from build123d import *

# Parameters (mm, degrees)
SKETCH1_W           = 20
SKETCH1_H           = 24
BOSS_EXTRUDE1_DEPTH = 8
SKETCH2_R           = 7
CUT_EXTRUDE1_DEPTH  = 22
BOSS_EXTRUDE2_DEPTH = 2


with BuildPart() as part:
    # Sketch1 → Boss-Extrude1 (new body)
    with BuildSketch(Plane(origin=(0, 0, 0), x_dir=(1, 0, 0), z_dir=(0, 1, 0))):
        Rectangle(SKETCH1_W, SKETCH1_H)
    extrude(amount=BOSS_EXTRUDE1_DEPTH)

    # Sketch2 → Cut-Extrude1 (cut)
    with BuildSketch(Plane.XY.offset(12)):
        Circle(SKETCH2_R)
    extrude(amount=-CUT_EXTRUDE1_DEPTH, mode=Mode.SUBTRACT)

    # Sketch3 → Boss-Extrude2 (add)
    with BuildSketch(Plane(origin=(0, 0, -12), x_dir=(-1, 0, 0), z_dir=(0, 0, -1))):
        with BuildLine():
            Line((-2, -6.708203932), (-2, -5))
            Line((-2, -5), (2, -5))
            Line((2, -5), (2, -6.708203932))
            ThreePointArc((2, -6.708203932), (0, 7), (-2, -6.708203932))
        make_face()
    extrude(amount=-BOSS_EXTRUDE2_DEPTH)


solid = part.part
Here's how the part is built. I have some questions about the finished solid (model axes, mm). A direction names the side the tool comes from. Coordinates: 2 decimals unless noted, no trailing zeros. Loops run counter-clockwise (first coordinate to the right, second up) from the corner with the lowest first, then second, coordinate; pieces in that order, holes last.
1. If we mould it in two halves opening along X, with no side actions, what happens to faces 1 (the flat face through (-9, 0, 0)), 2 (the flat face through (0, -5, -11)), 3 (the cylindrical face through (-5.6, -4.2, -11))? For each: pulls with the +X half, pulls with the -X half, needs draft (parallel to the pull), parting line crosses it, or undercut.
2. I need wall thicknesses on L1, parallel to Y at x = -8, z = 5; L2, parallel to Z at x = -6, y = 2.75; L3, parallel to Y at x = 0, z = -8.5. Which ranges of each line are inside material? Lowest first, please.
3. Imagine slicing it at B-B, the plane x = 0. Please give me the cut outline in (y, z), and give its area (3 significant figures).
4. For P1, Ø1.9, axis at y = -5.5, z = -11, coming from the -X side; P2, Ø2, axis at x = 0.5, z = -11, coming from the -Y side; P3, Ø0.9, axis at y = -6, z = -11.5, coming from the +X side, each with a flat end and sliding along its axis, tell me the tip position at first contact or that it passes through.
5. Imagine slicing it at A-A, the plane z = -2.5. Please give me the cut outline in (x, y).
6. Imagine slicing it at C-C, the plane x = -7.5. Please give me the cut outline in (y, z).
7. Imagine slicing it at D-D, the plane y = -2. Please give me the cut outline in (x, z).
8. For faces 4 (the flat face through (0, 8, 0)), 5 (the flat face through (-2, -6, -11)), 6 (the cylindrical face through (0, 7, 1)), which set-ups out of +Z, -Z, +X, -X, +Y, -Y let a thin tool reach every point of the face, with its end or its side?
Taken from the geometry:
1. face 1: needs draft
1. face 2: undercut
1. face 3: pulls with the -X half
2. L1: y = 0 to 8
2. L2: z = -12 to -10
2. L3: y = 7 to 8
3. outline: (-5, -12) - (8, -12) - (8, 12) - (7, 12) - (7, -10) - (-5, -10) - close
3. area: 48.0 mm2
4. P1: stops at x = -5.32
4. P2: stops at y = -5
4. P3: stops at x = 4.27
5. outline: (-10, 0) - (-7, 0) arc R7 cw to (7, 0) - (10, 0) - (10, 8) - (-10, 8) - close
6. outline: (0, -12) - (8, -12) - (8, 12) - (0, 12) - close
7. outline: (-6.71, -12) - (6.71, -12) - (6.71, -10) - (-6.71, -10) - close
8. face 4: +Z, -Z, +X, -X, +Y
8. face 5: +Z, -Z, -Y
8. face 6: +Z, -Y
